Geometry check sheet. Reference: the model listing, model coordinates, mm. Face numbers are marked on the shaded views. A direction names the side the tool comes from. Coordinates: 2 decimals unless noted, no trailing zeros. Write each loop counter-clockwise with the first axis right and the second up, starting at its lowest first coordinate (ties: lowest second). Pieces come first, ordered by that corner, then holes. Notation, with made-up numbers: M -35.75,-5 L 7.25,-5 A7 cw 7.25,3 Z; hole C 29,37 d2. An arc over 180 degrees is marked long. Put each result on its own line as item: value. Start each with the question number.
1) Cross-section at C-C on x = 13. Record the cut outline in (y, z).
2) Set-up check for the marked faces 3 and 4: record each of +Z, -Z, +X, -X, +Y, -Y from which the full face is reachable in a straight line by a thin tool's end or side.
3) Cross-section at B-B on x = -5.1. Record the cut outline in (y, z), plus the area to 3 significant figures.
4) Gauge pin test, flat ends, axial feed: pin 1 (0.8 mm diameter, centred on y = -1, z = 0.5, fed in from -X); pin 2 (1 mm diameter, centred on y = -13, z = -0.5, fed in from +X); pin 3 (0.8 mm diameter, centred on x = -34, z = 0.5, fed in from -Y). Record the tip position at first contact, or that the pin passes through.
5) Mould release check, pull along X, two halves, no side actions. Record for the marked faces 1 and 2: released by +X, released by -X, zero draft, split by the parting line, or undercut.
6) Cross-section at A-A on x = -22.7. Record the cut outline in (y, z), plus the area to 3 significant figures.
7) Scan lines: line 1 along Y through (x, z) = (-30.85, 0.3); line 2 along Y through (x, z) = (15, -2.6); line 3 along X through (y, z) = (-7, -1). Record each from-to range of solid material in increasing order.
8) Cross-section at D-D on x = 24. Record the cut outline in (y, z).
from build123d import *

# Parameters (mm, degrees)
EXTRUDE_1_DEPTH     = 10
SKETCH_2_R          = 0.4
CUT_EXTRUDE_1_DEPTH = 15.682716688
SKETCH_3_R          = 0.4
EXTRUDE_2_DEPTH     = 1
EXTRUDE_3_REACH     = 45.175
SKETCH_4_W          = 2.5
SKETCH_4_H          = 3
EXTRUDE_4_REACH     = 48.044
SKETCH_5_W          = 1.5
SKETCH_5_H          = 3
LOFT_START          = -4
LOFT_2_DEPTH        = 1.5
EXTRUDE_7_DEPTH     = 4
EXTRUDE_8_DEPTH     = 1.5
SKETCH_13_W         = 25.4
SKETCH_13_H         = 20.35
SKETCH_13_R         = 1.3
EXTRUDE_9_DEPTH     = 1.5
SKETCH_14_W         = 17.5
SKETCH_14_H         = 30
SKETCH_14_R         = 1.5
EXTRUDE_10_DEPTH    = 1.5


# Read off the part's stored shape, not the designer's step: the loft step
with BuildPart() as part:
    # Sketch 1 → Extrude 1 (new body)
    with BuildSketch(Plane(origin=(0, 0, 0), x_dir=(0, 0, -1), z_dir=(1, 0, 0))):
        Polygon((0, 0), (0, 2.50113593), (1, 2.50113593), (1, -0.14886407), (4, -0.14886407), (4, -10.32386407), (0, -10.32386407), (0, -6.32386407), (2.5, -6.32386407), (2.5, -1.14886407), (0, -1.14886407), align=None)
    extrude_1 = extrude(amount=EXTRUDE_1_DEPTH)

    # Sketch 2 → Cut-Extrude 1 (cut, through all)
    with BuildSketch(Plane(origin=(0, 0, -1), x_dir=(-1, 0, 0), z_dir=(0, 0, -1))):
        with Locations(Location((-5, 1.00113593, 0), (0, 0, 90))):
            Circle(SKETCH_2_R)
    cut_extrude_1 = extrude(amount=-CUT_EXTRUDE_1_DEPTH, mode=Mode.SUBTRACT)

    # Mirror 1: Extrude 1, Cut-Extrude 1 across plane
    add(extrude_1.mirror(Plane(origin=(10, -10.32386407, -4), x_dir=(0, 0, 1), z_dir=(0, 1, 0))))
    add(cut_extrude_1.mirror(Plane(origin=(10, -10.32386407, -4), x_dir=(0, 0, 1), z_dir=(0, 1, 0))), mode=Mode.SUBTRACT)

    # Sketch 5 → Extrude 4 (add, up to next)
    with BuildSketch(Plane(origin=(-29.6, 0, 0), x_dir=(0, 0, -1), z_dir=(1, 0, 0)), mode=Mode.PRIVATE) as extrude_4_sk1:
        with Locations((3.25, -6.80386407)):
            Rectangle(SKETCH_5_W, SKETCH_5_H)
    extrude_4_tool1 = extrude(extrude_4_sk1.sketch, amount=EXTRUDE_4_REACH, mode=Mode.PRIVATE) - part.part
    # Sketch 5 → Extrude 4 (add, up to next)
    with BuildSketch(Plane(origin=(-29.6, 0, 0), x_dir=(0, 0, -1), z_dir=(1, 0, 0)), mode=Mode.PRIVATE) as extrude_4_sk2:
        with Locations((3.25, -13.80386407)):
            Rectangle(SKETCH_5_W, SKETCH_5_H)
    extrude_4_tool2 = extrude(extrude_4_sk2.sketch, amount=EXTRUDE_4_REACH, mode=Mode.PRIVATE) - part.part


with BuildPart() as body_2:
    # Sketch 3 → Extrude 2 (new body)
    with BuildSketch(Plane.XY.offset(1)):
        Polygon((-32.1, -0.15386407), (-32.1, -3.35386407), (-36.1, -3.35386407), (-36.1, -6.35386407), (-32.1, -6.35386407), (-32.1, -14.25386407), (-36.1, -14.25386407), (-36.1, -17.25386407), (-32.1, -17.25386407), (-32.1, -20.45386407), (-29.6, -20.45386407), (-29.6, -0.15386407), align=None)
        with Locations((-30.85, -3.30386407)):
            Circle(SKETCH_3_R, mode=Mode.SUBTRACT)
        with Locations((-30.85, -17.30386407)):
            Circle(SKETCH_3_R, mode=Mode.SUBTRACT)
    extrude(amount=-EXTRUDE_2_DEPTH)

    # Sketch 4 → Extrude 3 (add, up to next)
    with BuildSketch(Plane(origin=(0, 0, -4), x_dir=(-1, 0, 0), z_dir=(0, 0, -1)), mode=Mode.PRIVATE) as extrude_3_sk1:
        with Locations((30.85, -6.80386407)):
            Rectangle(SKETCH_4_W, SKETCH_4_H)
    extrude_3_tool1 = extrude(extrude_3_sk1.sketch, amount=-EXTRUDE_3_REACH, mode=Mode.PRIVATE) - body_2.part
    # Sketch 4 → Extrude 3 (add, up to next)
    with BuildSketch(Plane(origin=(0, 0, -4), x_dir=(-1, 0, 0), z_dir=(0, 0, -1)), mode=Mode.PRIVATE) as extrude_3_sk2:
        with Locations((30.85, -13.80386407)):
            Rectangle(SKETCH_4_W, SKETCH_4_H)
    extrude_3_tool2 = extrude(extrude_3_sk2.sketch, amount=-EXTRUDE_3_REACH, mode=Mode.PRIVATE) - body_2.part
    add(extrude_3_tool1.solids().sort_by_distance((-30.85, -6.803864, -4))[0])
    add(extrude_3_tool2.solids().sort_by_distance((-30.85, -13.803864, -4))[0])


with BuildPart() as part_1:
    add(part.part)

    add(body_2.part)  # Extrude 4 merges body 2
    add(extrude_4_tool1.solids().sort_by_distance((-29.6, -6.803864, -3.25))[0])
    add(extrude_4_tool2.solids().sort_by_distance((-29.6, -13.803864, -3.25))[0])

    # Sketch 8 → Loft 1 section 0
    with BuildSketch(Plane(origin=(45.5, 0, 0), x_dir=(0, 0, -1), z_dir=(1, 0, 0))):
        with BuildLine():
            Line((2.5, -1.32386407), (4, -1.32386407))
            Line((4, -1.32386407), (4, -4.32386407))
            Line((4, -4.32386407), (2.5, -4.32386407))
            Line((2.5, -4.32386407), (2.5, -1.32386407))
        make_face()
    # Sketch 7 → Loft 1 section 1
    with BuildSketch(Plane(origin=(10, 0, 0), x_dir=(0, 0, -1), z_dir=(1, 0, 0))):
        with BuildLine():
            Line((2.5, -5.30386407), (4, -5.30386407))
            Line((4, -5.30386407), (4, -8.30386407))
            Line((4, -8.30386407), (2.5, -8.30386407))
            Line((2.5, -8.30386407), (2.5, -5.30386407))
        make_face()
    loft()

    # Loft 2 outline → Loft 2 (add)
    with BuildSketch(Plane.XY.offset(LOFT_START)):
        Polygon((10, -15.30386407), (45.5, -19.32386407), (45.5, -16.32386407), (10, -12.30386407), align=None)
    extrude(amount=LOFT_2_DEPTH)

    # Sketch 11 → Extrude 7 (add)
    with BuildSketch(Plane(origin=(0, 0, -4), x_dir=(-1, 0, 0), z_dir=(0, 0, -1))):
        Polygon((-45.5, -1.32386407), (-44, -1.492033084), (-44, -4.492033084), (-45.5, -4.32386407), align=None)
        Polygon((-45.5, -16.32386407), (-45.5, -19.32386407), (-44, -19.154004915), (-44, -16.154004915), align=None)
    extrude(amount=-EXTRUDE_7_DEPTH)

    # Sketch 12 → Extrude 8 (add)
    with BuildSketch(Plane(origin=(0, 0, -4), x_dir=(-1, 0, 0), z_dir=(0, 0, -1))):
        Polygon((-30, -6.061610549), (-33, -5.725272521), (-33, -14.908371112), (-30, -14.568652803), align=None)
    extrude(amount=-EXTRUDE_8_DEPTH)

    # Sketch 13 → Extrude 9 (add)
    with BuildSketch(Plane(origin=(0, 0, -4), x_dir=(-1, 0, 0), z_dir=(0, 0, -1))):
        with Locations((-5, -10.32386407)):
            Rectangle(SKETCH_13_W, SKETCH_13_H)
        with Locations(Location((-15.1, -2.75386407, 0), (0, 0, 90))):
            Circle(SKETCH_13_R, mode=Mode.SUBTRACT)
        with Locations(Location((5.1, -2.75386407, 0), (0, 0, 270))):
            Circle(SKETCH_13_R, mode=Mode.SUBTRACT)
        with Locations(Location((5.1, -17.85386407, 0), (0, 0, 90))):
            Circle(SKETCH_13_R, mode=Mode.SUBTRACT)
        with Locations(Location((-15.1, -17.85386407, 0), (0, 0, 270))):
            Circle(SKETCH_13_R, mode=Mode.SUBTRACT)
    extrude(amount=-EXTRUDE_9_DEPTH)

    # Sketch 14 → Extrude 10 (add)
    with BuildSketch(Plane(origin=(0, 0, -4), x_dir=(-1, 0, 0), z_dir=(0, 0, -1))):
        with Locations((16.45, -10.30386407)):
            Rectangle(SKETCH_14_W, SKETCH_14_H)
        with Locations(Location((22.7, -22.80386407, 0), (0, 0, 90))):
            Circle(SKETCH_14_R, mode=Mode.SUBTRACT)
    extrude(amount=-EXTRUDE_10_DEPTH)


solid = part_1.part
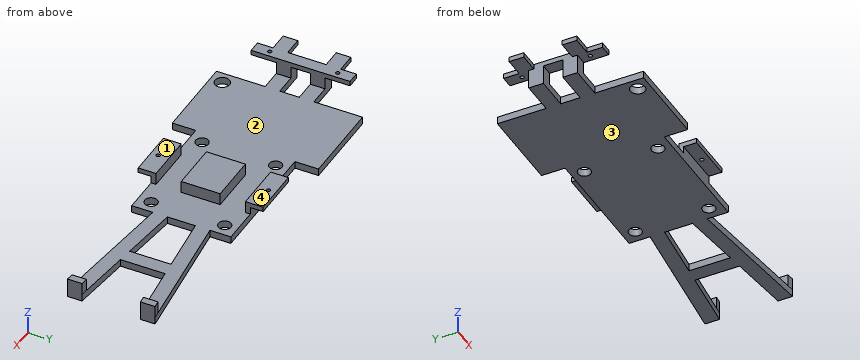
Answer key:
1. outline: M -20.5,-4 L -0.15,-4 L -0.15,-2.5 L -20.5,-2.5 Z
2. face 3: -Z, +X, -X, +Y, -Y
2. face 4: +Z, +X, +Y, -Y
3. outline: M -20.5,-4 L -19.15,-4 L -19.15,-2.5 L -20.5,-2.5 Z; M -16.55,-4 L -4.05,-4 L -4.05,-2.5 L -16.55,-2.5 Z; M -1.45,-4 L -0.15,-4 L -0.15,-2.5 L -1.45,-2.5 Z
3. area: 22.7 mm²
4. pin 1: stops at x = -32.1
4. pin 2: stops at x = 10
4. pin 3: stops at y = -17.25
5. face 1: zero draft
5. face 2: undercut
6. outline: M -25.3,-4 L -24.3,-4 L -24.3,-2.5 L -25.3,-2.5 Z; M -21.3,-4 L 4.7,-4 L 4.7,-2.5 L -21.3,-2.5 Z
6. area: 40.5 mm²
7. line 1: y = -20.45 to -17.7, -16.9 to -3.7, -2.9 to -0.15
7. line 2: y = -20.5 to -19.15, -16.56 to -4.05, -1.46 to -0.15
7. line 3: x = -32.1 to -29.6, 0 to 10
8. outline: M -16.89,-4 L -13.89,-4 L -13.89,-2.5 L -16.89,-2.5 Z; M -6.73,-4 L -3.73,-4 L -3.73,-2.5 L -6.73,-2.5 Z
